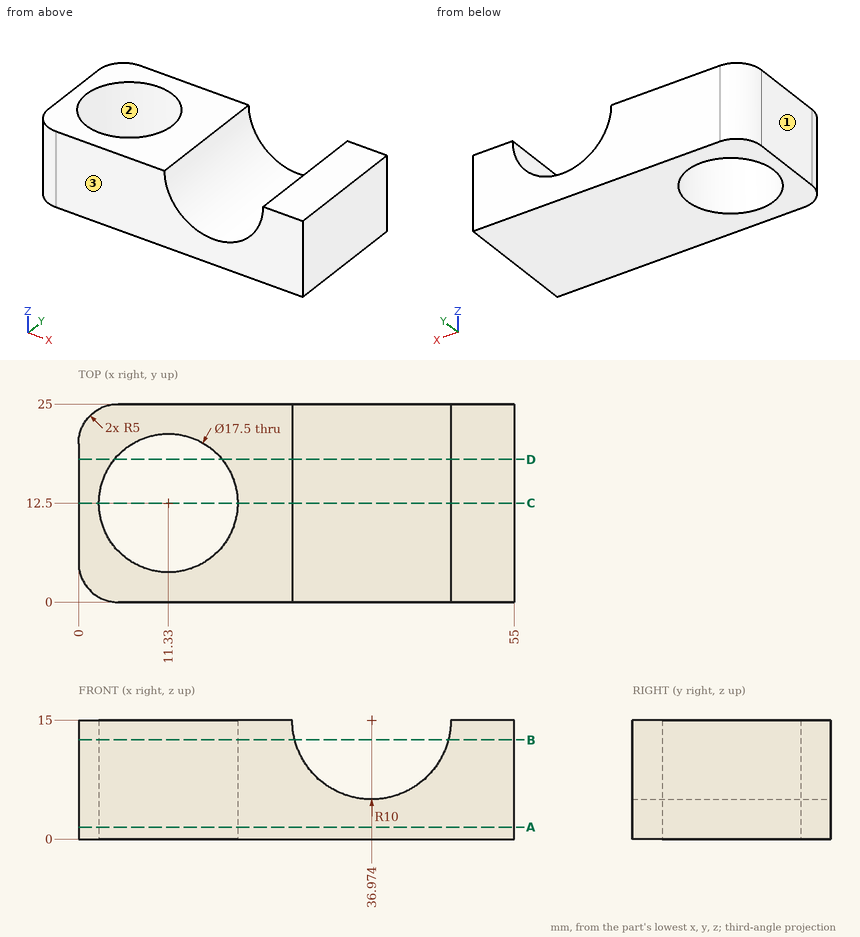
Job drawing, mm, ordinate dimensions from the low corner. One solid piece. Coordinates: 2 decimals unless noted, no trailing zeros. Order: outer loops, then holes, each group sorted by start corner. A loop starts at its lowest first (then second) coordinate and runs counter-clockwise, first axis right, second up. Notation, with made-up numbers: (83, -18) -> (91, -18) arc R16 cw to (91, 3) -> close; hole circle Ø5 at (-32, 5.25). An arc over 180 degrees is marked (long way). Answer in a Markdown table with one row per item. Add a question column.
Q1. Band-saw the part on D-D, the plane y = 18. List the corners of the cut face in (x, z) (1 decimal).
Q2. Mould opens along Y. For the marked faces 1, 2 and 3 say: +Y half, -Y half, draft (parallel to the pull), parting line (faces both ways), or undercut.
Q3. Band-saw the part on B-B, the plane z = 12.5. List the corners of the cut face in (x, y).
Q4. Wall check: line 1 along X through (y, z) = (19.75, 7) (1 decimal); line 2 along Y through (x, z) = (4, 1.5); line 3 along Y through (x, z) = (17.5, 1.5) (1 decimal). Give the ranges that are in metal, low to high. Write a range as [from, to].
Q5. Drop a flat-ended pin along its axis: pin 1 (8 mm diameter, centred on y = 7.5, z = 3, fed in from -X). Give the stop position or say it passes through.
Q6. Band-saw the part on C-C, the plane y = 12.5. List the corners of the cut face in (x, z).
Q7. Band-saw the part on A-A, the plane z = 1.5. List the corners of the cut face in (x, y).
Answers follow:
| question | item | result |
|---|---|---|
| 1 | outline | (0, 0) -> (4.5, 0) -> (4.5, 15) -> (0, 15) -> close; (18.1, 0) -> (55, 0) -> (55, 15) -> (47, 15) arc R10 cw to (27, 15) -> (18.1, 15) -> close |
| 2 | face 1 | draft |
| 2 | face 2 | undercut |
| 2 | face 3 | -Y half |
| 3 | outline | (0, 5) arc R5 ccw to (5, 0) -> (27.29, 0) -> (27.29, 25) -> (5, 25) arc R5 ccw to (0, 20) -> close; (46.66, 0) -> (55, 0) -> (55, 25) -> (46.66, 25) -> close; hole circle Ø17.5 at (11.33, 12.5) |
| 4 | line 1 | [0, 6.4], [16.2, 31], [43, 55] |
| 4 | line 2 | [0.1, 7.72], [17.28, 24.9] |
| 4 | line 3 | [0, 6.3], [18.7, 25] |
| 5 | pin 1 | x = 0 |
| 6 | outline | (0, 0) -> (2.58, 0) -> (2.58, 15) -> (0, 15) -> close; (20.08, 0) -> (55, 0) -> (55, 15) -> (46.97, 15) arc R10 cw to (26.97, 15) -> (20.08, 15) -> close |
| 7 | outline | (0, 5) arc R5 ccw to (5, 0) -> (55, 0) -> (55, 25) -> (5, 25) arc R5 ccw to (0, 20) -> close; hole circle Ø17.5 at (11.33, 12.5) |
